Source: CAD feature listing. Evaluate the final solid. Frame: model axes, mm. A direction names the side the tool comes from. Give positions to 0.01 mm unless a question says otherwise; leave off trailing zeros. Order: outer loops, then holes, each group sorted by start corner. A loop starts at its lowest first (then second) coordinate and runs counter-clockwise, first axis right, second up.
from build123d import *

# Parameters (mm, degrees)
SKETCH_1_W          = 100
SKETCH_1_H          = 50
EXTRUDE_1_DEPTH     = 40
SKETCH_2_W          = 60
SKETCH_2_H          = 17.5
CUT_EXTRUDE_1_DEPTH = 70
SKETCH_4_R          = 1.3
CUT_EXTRUDE_2_DEPTH = 119.74342087
EXTRUDE_2_DEPTH     = 50
SKETCH_6_R          = 10
CUT_EXTRUDE_3_DEPTH = 278.729911697
SKETCH_7_R          = 1.3
CUT_EXTRUDE_4_DEPTH = 278.740409113
FILLET_1_R          = 10
FILLET_2_R          = 1


with BuildPart() as part:
    # 草圖1 → 填料-伸長1 (new body)
    with BuildSketch(Plane.XY):
        with Locations((50, 25)):
            Rectangle(SKETCH_1_W, SKETCH_1_H)
    extrude(amount=EXTRUDE_1_DEPTH)

    # 草圖2 → 除料-伸長1 (cut)
    with BuildSketch(Plane.XY.offset(40)):
        with Locations((43, 33.75)):
            Rectangle(SKETCH_2_W, SKETCH_2_H)
        with Locations((43, 16.25)):
            Rectangle(SKETCH_2_W, SKETCH_2_H)
    extrude(amount=-CUT_EXTRUDE_1_DEPTH, mode=Mode.SUBTRACT)

    # 草圖4 → 除料-伸長2 (cut, through all)
    with BuildSketch(Plane(origin=(0, 50, 0), x_dir=(1, 0, 0), z_dir=(0, 1, 0))):
        with Locations(Location((43, -36.6, 0), (0, 0, 270))):
            Circle(SKETCH_4_R)
    extrude(amount=-CUT_EXTRUDE_2_DEPTH, mode=Mode.SUBTRACT)

    # 草圖5 → 填料-伸長2 (add)
    with BuildSketch(Plane(origin=(0, 50, 0), x_dir=(1, 0, 0), z_dir=(0, 1, 0))):
        Polygon((149.133929878, -46.468604585), (100, -40), (100, 0), (159.486691682, -7.831571533), (262.937008695, -35.551000434), (252.584246891, -74.188033485), align=None)
    extrude(amount=-EXTRUDE_2_DEPTH)

    # 草圖6 → 除料-伸長3 (cut, through all)
    with BuildSketch(Plane(origin=(-1.627072127, 0, 6.072315847), x_dir=(0.9659258262890664, 0, 0.2588190451025279), z_dir=(-0.25881904510252796, 0, 0.9659258262890664))):
        with Locations((230.147023393, 25)):
            Circle(SKETCH_6_R)
    extrude(amount=-CUT_EXTRUDE_3_DEPTH, mode=Mode.SUBTRACT)

    # 草圖7 → 除料-伸長4 (cut, through all)
    with BuildSketch(Plane(origin=(0, 50, 0), x_dir=(1, 0, 0), z_dir=(0, 1, 0))):
        with Locations(Location((221.713157792, -61.77504537, 0), (0, 0, 270))):
            Circle(SKETCH_7_R)
    extrude(amount=-CUT_EXTRUDE_4_DEPTH, mode=Mode.SUBTRACT)

    # 圓角1
    fillet_1_edges = [part.edges().sort_by_distance(p)[0] for p in [
        (257.760627793, 0, 54.869516959),
        (257.760627793, 50, 54.869516959),
        (0, 50, 20),
        (0, 0, 20),
    ]]
    fillet(fillet_1_edges, radius=FILLET_1_R)

    # 圓角2
    fillet_2_edges = [part.edges().sort_by_distance(p)[0] for p in [
        (55, 50, 40),
        (43, 7.5, 0),
        (73, 25, 0),
        (43, 42.5, 0),
        (13, 25, 0),
        (43, 42.5, 40),
        (73, 25, 40),
        (13, 25, 40),
        (43, 7.5, 40),
        (196.029459253, 0, 59.034223809),
        (206.382221057, 50, 20.397190758),
        (129.743345841, 0, 3.915785767),
        (129.743345841, 50, 3.915785767),
        (124.566964939, 0, 43.234302292),
        (124.566964939, 50, 43.234302292),
        (55, 50, 0),
        (211.018623349, 25, 63.050558224),
        (252.584246891, 25, 74.188033485),
        (262.937008695, 25, 35.551000434),
        (196.029459253, 50, 59.034223809),
        (249.755115647, 2.928932188, 73.429970053),
        (249.755115647, 47.071067812, 73.429970053),
        (206.382221057, 0, 20.397190758),
        (260.107877451, 2.928932188, 34.792937001),
        (260.107877451, 47.071067812, 34.792937001),
        (55, 0, 0),
        (55, 0, 40),
        (0, 25, 0),
        (0, 25, 40),
        (2.928932188, 2.928932188, 0),
        (2.928932188, 47.071067812, 0),
        (2.928932188, 2.928932188, 40),
        (2.928932188, 47.071067812, 40),
    ]]
    fillet(fillet_2_edges, radius=FILLET_2_R)


solid = part.part
(1) Access query for faces 1 (the cylindrical face through (130.121, 0.285, 4.269)), 2 (the flat face through (13, 25, 20)), 3 (the flat face through (61, 47, 40)). Directions: +Z, -Z, +X, -X, +Y, -Y. A direction counts if a zero-diameter tool reaches every point of the face in a straight line with its end or side. Return the directions, or none.
(2) Section B-B, the plane x = 76.5. Return loops of the section in (y, z), plus the area to 3 significant figures.
(3) Pin query (flat end, axial travel): pin 1 Ø2 at (x, z) = (43, 36.6) entering from -Y; pin 2 Ø3 at (x, y) = (214, 32.5) entering from -Z; pin 3 Ø2 at (x, y) = (121.5, 22.5) entering from -Z; pin 4 Ø8 at (x, y) = (107, 35) entering from +Z. Return the tip coordinate at first contact, or that it passes through.
(4) Section A-A, the plane x = 18. Return loops of the section in (y, z).
(5) Line query: line 1 along Y through (x, z) = (36, 29); line 2 along X through (y, z) = (47, 36); line 3 along X through (y, z) = (45.75, 36.6). Output: solid intervals per line, ascending.
(6) Draft query along Y for faces 4 (the flat face through (43, 7.5, 20)), 5 (the flat face through (61, 47, 0)), 6 (the flat face through (43, 42.5, 20)), 7 (the cylindrical face through (3.01, 47.15, 20.27)). Return one class per face: +Y half, -Y half, draft (parallel to the pull), parting line (faces both ways), or undercut.
Checks:
1. face 1: -Z, +X, -Y
1. face 2: +Z, -Z
1. face 3: +Z, -X, +Y, -Y
2. outline: (0, 1) arc R1 ccw to (1, 0) - (49, 0) arc R1 ccw to (50, 1) - (50, 39) arc R1 ccw to (49, 40) - (1, 40) arc R1 ccw to (0, 39) - close
2. area: 2,000 mm2
3. pin 1: passes through
3. pin 2: stops at z = 22.04
3. pin 3: stops at z = 2.7
3. pin 4: stops at z = 41.45
4. outline: (0, 1) arc R1 ccw to (1, 0) - (6.5, 0) arc R1 ccw to (7.5, 1) - (7.5, 39) arc R1 ccw to (6.5, 40) - (1, 40) arc R1 ccw to (0, 39) - close; (42.5, 1) arc R1 ccw to (43.5, 0) - (49, 0) arc R1 ccw to (50, 1) - (50, 39) arc R1 ccw to (49, 40) - (43.5, 40) arc R1 ccw to (42.5, 39) - close
5. line 1: y = 0 to 7.5, 42.5 to 50
5. line 2: x = 2.86 to 41.85, 44.15 to 259.86
5. line 3: x = 1.82 to 41.7, 44.3 to 260.77
6. face 4: undercut
6. face 5: draft
6. face 6: undercut
6. face 7: +Y half
